Read the model definition and answer for the solid it produces. Units are mm, in the model's axes. Face numbers are marked on the shaded views. A direction names the side the tool comes from. Coordinates: 2 decimals unless noted, no trailing zeros. Loops run counter-clockwise (first coordinate to the right, second up) from the corner with the lowest first, then second, coordinate; pieces in that order, holes last. Notation, with made-up numbers: (-12.75, 87.5) - (39.25, 87.5) arc R24 cw to (39.25, 105.5) - close; hole circle Ø3 at (4, -25). An arc over 180 degrees is marked (long way). One line per question, with ' | ' between items. Start each with the question number.
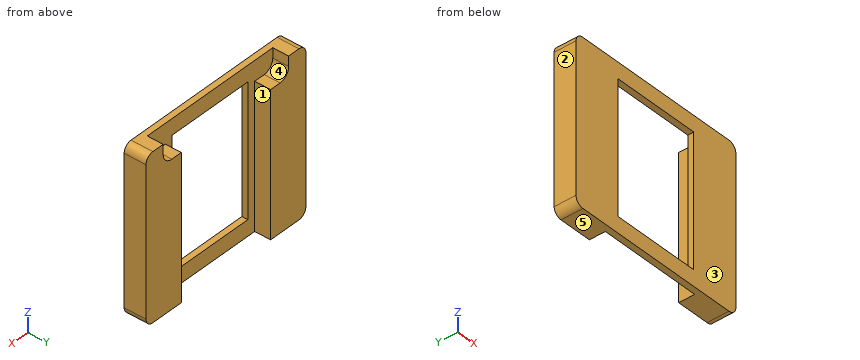
Autodesk Fusion 360 part; units mm, degrees
sketch "Sketch1" plane through (0, 0, 0) normal (0, 1, 0) x (1, 0, 0)
  line L0 (23.25, 20.5) -> (-23.25, 20.5)
  line L1 (-23.25, 20.5) -> (-23.25, -20.5)
  line L2 (-23.25, -20.5) -> (23.25, -20.5)
  line L3 (23.25, -20.5) -> (23.25, 20.5)
  line L4 (23.25, 20.5) -> (-23.25, -20.5) construction
  line L5 (-23.25, 20.5) -> (23.25, -20.5) construction
  dimension "d1" = 46.5
  dimension "d2" = 41
extrude "Extrude1" add sketch "Sketch1" along normal blind 5.5
sketch "Sketch2" plane through (0, 5.5, 0) normal (0, 1, 0) x (-1, 0, 0)
  line L0 (-23.25, 20.5) -> (-23.25, -20.5)
  line L1 (-23.25, -20.5) -> (23.25, -20.5)
  line L2 (23.25, -20.5) -> (23.25, 20.5)
  line L3 (23.25, 20.5) -> (-23.25, 20.5)
  line L4 (-13, -20.5) -> (13, -20.5)
  line L5 (13, -20.5) -> (13, 20.5)
  line L6 (13, 20.5) -> (-13, 20.5)
  line L7 (-13, 20.5) -> (-13, -20.5)
  line L8 (-13, -20.5) -> (13, 20.5) construction
  line L9 (13, -20.5) -> (-13, 20.5) construction
  line L10 (18.25, 20.5) -> (-18.25, 20.5)
  line L11 (-18.25, 20.5) -> (-18.25, 15.5)
  line L12 (-18.25, 15.5) -> (18.25, 15.5)
  line L13 (18.25, 15.5) -> (18.25, 20.5)
  dimension "d5" = 26
  dimension "d6" = 5
  dimension "d7" = 5
  dimension "d8" = 5
extrude "Extrude2" cut sketch "Sketch2" against normal blind 4 contours L3 L7 L10 L11 L12 | L1 L4 L5 L7 L12 | L3 L5 L6 L7 L10 L12 | L3 L5 L10 L12 L13
fillet "Fillet1" radius 2.5 1 edges at (-18.25, 3.5, 15.5)
fillet "Fillet1" radius 2.5 1 edges at (18.25, 3.5, 15.5)
sketch "Sketch3" plane through (0, 1.5, 0) normal (0, 1, 0) x (-1, 0, 0)
  arc A0 (-18.25, 18) -> (-15.75, 15.5) centre (-15.75, 18) ccw
  line L0 (-15.75, 15.5) -> (-13, 15.5)
  line L1 (-13, 15.5) -> (-13, -20.5)
  line L2 (-13, -20.5) -> (13, -20.5)
  line L3 (13, -20.5) -> (13, 15.5)
  line L4 (13, 15.5) -> (15.75, 15.5)
  arc A1 (15.75, 15.5) -> (18.25, 18) centre (15.75, 18) ccw
  line L5 (18.25, 18) -> (18.25, 20.5)
  line L6 (18.25, 20.5) -> (-18.25, 20.5)
  line L7 (-18.25, 20.5) -> (-18.25, 18)
  line L8 (11, -16.5) -> (-11, -16.5)
  line L9 (-11, -16.5) -> (-11, 16.5)
  line L10 (-11, 16.5) -> (11, 16.5)
  line L11 (11, 16.5) -> (11, -16.5)
  dimension "d15" = 2
  dimension "d16" = 2
  dimension "d17" = 4
  dimension "d18" = 4
extrude "Extrude3" cut sketch "Sketch3" against normal blind 2 contours L8 L9 L10 L11
fillet "Fillet2" radius 2 1 edges at (-23.25, 2.75, 20.5)
fillet "Fillet2" radius 2 1 edges at (23.25, 2.75, 20.5)
fillet "Fillet2" radius 2 1 edges at (23.25, 2.75, -20.5)
fillet "Fillet2" radius 2 1 edges at (-23.25, 2.75, -20.5)
1) The mould has two halves that part along X. Classify the marked faces 1, 2 and 3: released by +X, released by -X, zero draft, split by the parting line, or undercut.
2) The part is cut by section D-D on x = 8. Write down the section's boundary in (y, z).
3) The part is cut by section A-A on z = 16. Write down the section's boundary in (x, y), and give its area (4 significant figures).
4) The part is cut by section B-B on y = 0.7. Write down the section's boundary in (x, z).
5) The part is cut by section C-C on y = 4.6. Write down the section's boundary in (x, z).
6) Given pin 1 Ø3 at (x, y) = (15, 3.5) entering from +Z; pin 2 Ø3 at (x, y) = (-14.5, 4) entering from +Z, each flat-ended and moving along its own axis, determine where each tip first touches the part or whether it passes through.
7) Which of the six approach directions +Z, -Z, +X, -X, +Y, -Y give full straight-line access (tool end or side, diameter ignored) to the marked faces 4 and 5?
8) Find the intervals of material crossed by line 1 along X through (y, z) = (0.3, 5.5); line 2 along X through (y, z) = (3, -17); line 3 along Z through (x, y) = (3, 0.4), in increasing order. Write a range as from..to.
Answer below:
1) face 1: undercut | face 2: released by -X | face 3: zero draft
2) outline: (0, -20.5) - (1.5, -20.5) - (1.5, -16.5) - (0, -16.5) - close; (0, 16.5) - (1.5, 16.5) - (1.5, 20.5) - (0, 20.5) - close
3) outline: (-23.25, 0) - (-11, 0) - (-11, 1.5) - (-17.25, 1.5) - (-17.25, 5.5) - (-23.25, 5.5) - close; (11, 0) - (23.25, 0) - (23.25, 5.5) - (17.25, 5.5) - (17.25, 1.5) - (11, 1.5) - close | area: 84.75 mm2
4) outline: (-23.25, -18.5) arc R2 ccw to (-21.25, -20.5) - (21.25, -20.5) arc R2 ccw to (23.25, -18.5) - (23.25, 18.5) arc R2 ccw to (21.25, 20.5) - (-21.25, 20.5) arc R2 ccw to (-23.25, 18.5) - close; hole (-11, -16.5) - (11, -16.5) - (11, 16.5) - (-11, 16.5) - close
5) outline: (-23.25, -18.5) arc R2 ccw to (-21.25, -20.5) - (-13, -20.5) - (-13, 15.5) - (-15.75, 15.5) arc R2.5 cw to (-18.25, 18) - (-18.25, 20.5) - (-21.25, 20.5) arc R2 ccw to (-23.25, 18.5) - close; (13, -20.5) - (21.25, -20.5) arc R2 ccw to (23.25, -18.5) - (23.25, 18.5) arc R2 ccw to (21.25, 20.5) - (18.25, 20.5) - (18.25, 18) arc R2.5 cw to (15.75, 15.5) - (13, 15.5) - close
6) pin 1: z = 15.62 | pin 2: z = 15.51
7) face 4: +Z, +Y | face 5: -Z, +X, -X, +Y, -Y
8) line 1: -23.25..-11, 11..23.25 | line 2: -23.25..-13, 13..23.25 | line 3: -20.5..-16.5, 16.5..20.5
